from build123d import *

# Parameters (mm, degrees)
SKETCH1_R           = 7.5
SKETCH1_W           = 3.175
SKETCH1_H           = 12.7
BOSS_EXTRUDE1_DEPTH = 3.175


with BuildPart() as part:
    # Sketch1 → Boss-Extrude1 (new body)
    with BuildSketch(Plane(origin=(0, 0, 0), x_dir=(1, 0, 0), z_dir=(0, 1, 0))):
        Polygon((0, 0), (15.302420881, 0), (15.302420881, -3.175), (28.002420881, -3.175), (28.002420881, 0), (53.402420881, 0), (53.402420881, -3.175), (66.102420881, -3.175), (66.102420881, 0), (81.404841762, 0), (81.404841762, 19.05), (81.404841762, 38.1), (81.404841762, 57.15), (66.102420881, 57.15), (66.102420881, 60.325), (53.402420881, 60.325), (53.402420881, 57.15), (28.002420881, 57.15), (28.002420881, 60.325), (15.302420881, 60.325), (15.302420881, 57.15), (0, 57.15), (-3.175, 57.15), (-3.175, 0), align=None)
        with Locations(Location((68.704841762, 28.575, 0), (0, 0, 270))):
            Circle(SKETCH1_R, mode=Mode.SUBTRACT)
        with Locations((47.3075, 15.875)):
            Rectangle(SKETCH1_W, SKETCH1_H, mode=Mode.SUBTRACT)
        with Locations((47.3075, 41.275)):
            Rectangle(SKETCH1_W, SKETCH1_H, mode=Mode.SUBTRACT)
        Polygon((26.350084324, 29.310366676), (31.353146576, 17.637347868), (34.271401278, 18.888113431), (29.268339026, 30.561132239), align=None, mode=Mode.SUBTRACT)
        Polygon((17.153101684, 21.678911781), (26.350084324, 12.920743576), (28.539626376, 15.219989236), (19.342643735, 23.978157441), align=None, mode=Mode.SUBTRACT)
        Polygon((12.270885661, 10.90317475), (13.382794097, 13.87710895), (25.2785309, 9.429475209), (24.166622465, 6.455541008), align=None, mode=Mode.SUBTRACT)
    extrude(amount=BOSS_EXTRUDE1_DEPTH)


solid = part.part
Can you work these out from the model? Positions are in its coordinate system, mm. A direction names the side the tool comes from. Coordinates: 2 decimals unless noted, no trailing zeros. Write each loop counter-clockwise with the first axis right and the second up, starting at its lowest first coordinate (ties: lowest second). Pieces come first, ordered by that corner, then holes.
Q1. Which directions (+Z, -Z, +X, -X, +Y, -Y) give clear straight access to the entire face, cutting with the end or side of a thin tool? Please do faces 1 (the face through (28.002, 2, -59)), 2 (the face through (22, 2, -60.325)), 3 (the face through (6, 2, -57.15)), 4 (the face through (47, 2, -47.625)), 5 (the face through (74, 2, 0)).
Results found:
face 1: -Z, +Y, -Y
face 2: -Z, +X, -X, +Y, -Y
face 3: -Z, -X, +Y, -Y
face 4: +Y, -Y
face 5: +Z, +X, +Y, -Y
Q2. Imagine slicing it at B-B, the plane z = -26.5. List the corners of the cut face in (x, y) for me (3 decimals).
Results found:
outline: (-3.175, 0) - (27.555, 0) - (27.555, 3.175) - (-3.175, 3.175) - close; (31.009, 0) - (61.498, 0) - (61.498, 3.175) - (31.009, 3.175) - close; (75.912, 0) - (81.405, 0) - (81.405, 3.175) - (75.912, 3.175) - close
Q3. Imagine slicing it at D-D, the plane y = 1.5. Count the separate pieces of the cut face and the enclosed holes in it, plus the area to 3 significant figures.
Results found:
separate pieces: 1
enclosed holes: 6
area: 4,620 mm2
Q4. For P1, Ø1, axis at y = 1, z = 1, coming from the -X side; P2, Ø1.6, axis at x = 46.5, y = 2, coming from the +Z side; P3, Ø1, axis at x = 11, y = 1, coming from the -Z side, each with a flat end and sliding along its axis, tell me the tip position at first contact or that it passes through.
Results found:
P1: stops at x = 15.3
P2: stops at z = 0
P3: stops at z = -57.15
Q5. Imagine slicing it at C-C, the plane x = 64.5. List the corners of the cut face in (y, z) for me (3 decimals), plus the area to 3 significant figures.
Results found:
outline: (0, -60.325) - (3.175, -60.325) - (3.175, -34.785) - (0, -34.785) - close; (0, -22.365) - (3.175, -22.365) - (3.175, 3.175) - (0, 3.175) - close
area: 162 mm2
Q6. Imagine slicing it at A-A, the plane z = -41.5. List the corners of the cut face in (x, y) for me (3 decimals).
Results found:
outline: (-3.175, 0) - (45.72, 0) - (45.72, 3.175) - (-3.175, 3.175) - close; (48.895, 0) - (81.405, 0) - (81.405, 3.175) - (48.895, 3.175) - close
Q7. Please list where these lines run through material, in increasing order: L1, parallel to Z at x = 46, y = 0.9 (3 decimals); L2, parallel to X at y = 2.05, z = -44 (3 decimals); L3, parallel to X at y = 1.75, z = -26 (3 decimals).
Results found:
L1: z = -57.15 to -47.625, -34.925 to -22.225, -9.525 to 0
L2: x = -3.175 to 45.72, 48.895 to 81.405
L3: x = -3.175 to 27.769, 31.223 to 61.661, 75.749 to 81.405
Q8. If we mould it in two halves opening along X, with no side actions, what happens to faces 6 (the face through (60, 2, -60.325)), 7 (the face through (27.83, 1.565, -29.945)), 8 (the face through (15.302, 2, 2))? For each: +X half, -X half, draft (parallel to the pull), parting line (faces both ways), or undercut.
Results found:
face 6: draft
face 7: undercut
face 8: -X half
